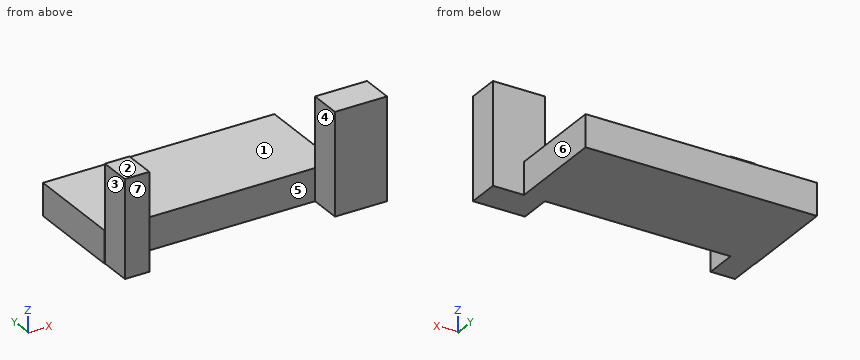
from build123d import *

# Parameters (mm, degrees)
F0_W     = 182.7251240611
F0_H     = 78.556381166
F1_DEPTH = 25.4
F2_W     = 19.2864239216
F2_H     = 76.4613673091
F3_DEPTH = 25.4
F4_W     = 15.6851392239
F4_H     = 80.182261765
F5_DEPTH = 25.4
F6_DEPTH = 25.4


with BuildPart() as f1:
    # F0 (on Top) → F1 (new body)
    with BuildSketch(Plane.XY):
        with Locations((-55.9463985264, 39.278190583)):
            Rectangle(F0_W, F0_H)
    extrude(amount=F1_DEPTH)

    # F2 (on Front) → F3 (join)
    with BuildSketch(Plane.XZ):
        with Locations((-137.3333185911, 38.2306836545)):
            Rectangle(F2_W, F2_H)
    extrude(amount=F3_DEPTH)

    # F4 (on Front) → F5 (join)
    with BuildSketch(Plane.XZ):
        with Locations((26.723430492, 40.0911308825)):
            Rectangle(F4_W, F4_H)
    extrude(amount=F5_DEPTH)

    # F6 (add): a face of the model
    f6_faces = [f1.faces().sort_by_distance(p)[0] for p in [
        (34.566000104, -12.7, 40.0911308825),
    ]]
    extrude(f6_faces, amount=F6_DEPTH)


solid = f1.part
Geometry check sheet. Reference: the model listing, model coordinates, mm. Face numbers are marked on the shaded views. A direction names the side the tool comes from. Round coordinates to 2 decimals unless told otherwise and drop trailing zeros. Order: outer loops, then holes, each group sorted by start corner. A loop starts at its lowest first (then second) coordinate and runs counter-clockwise, first axis right, second up. Notation, with made-up numbers: (37.25, 65) -> (65.25, 65) arc R17 ccw to (65.25, 90) -> close; hole circle Ø9 at (-22, 52.25). An arc over 180 degrees is marked (long way). Use one line per item in the form item = value.
1. Cross-section at C-C, the plane x = 22.5. Enter the section's corners in (y, z).
Working result:
outline = (-25.4, 0) -> (78.56, 0) -> (78.56, 25.4) -> (0, 25.4) -> (0, 80.18) -> (-25.4, 80.18) -> close
2. Go/stop test with flat-tipped pins: pin 1 (20.5 mm diameter, centred on y = -15, z = 42.5, fed in from -X); pin 2 (12.5 mm diameter, centred on y = 47, z = 12, fed in from +X); pin 3 (6 mm diameter, centred on x = -134, z = 55.5, fed in from +Y). Record where each tip stops, or that it passes through.
Working result:
pin_1 = -146.98
pin_2 = 35.42
pin_3 = 0
3. Cross-section at B-B, the plane y = -2. Enter the section's corners in (x, z), plus the area to 3 significant figures.
Working result:
outline = (-146.98, 0) -> (-127.69, 0) -> (-127.69, 76.46) -> (-146.98, 76.46) -> close; (18.88, 0) -> (59.97, 0) -> (59.97, 80.18) -> (18.88, 80.18) -> close
area = 4,770 mm^2
4. Mould release check, pull along X, two halves, no side actions. Record for the marked faces 5, 6 and 7: pulls with the +X half, pulls with the -X half, needs draft (parallel to the pull), parting line crosses it, or undercut.
Working result:
face_5 = undercut
face_6 = pulls with the +X half
face_7 = needs draft
5. Cross-section at A-A, the plane z = 40.5. Enter the section's corners in (x, y), plus the area to 3 significant figures.
Working result:
outline = (-146.98, -25.4) -> (-127.69, -25.4) -> (-127.69, 0) -> (-146.98, 0) -> close; (18.88, -25.4) -> (59.97, -25.4) -> (59.97, 0) -> (18.88, 0) -> close
area = 1,530 mm^2
6. Cross-section at D-D, the plane z = 9. Enter the section's corners in (x, y).
Working result:
outline = (-147.31, 0) -> (-146.98, 0) -> (-146.98, -25.4) -> (-127.69, -25.4) -> (-127.69, 0) -> (18.88, 0) -> (18.88, -25.4) -> (59.97, -25.4) -> (59.97, 0) -> (35.42, 0) -> (35.42, 78.56) -> (-147.31, 78.56) -> close
7. Set-up check for the marked faces 1, 2, 3 and 4: record each of +Z, -Z, +X, -X, +Y, -Y from which the full face is reachable in a straight line by a thin tool's end or side.
Working result:
face_1 = +Z, +X, -X, +Y
face_2 = +Z, -X, +Y, -Y
face_3 = +Z, -Z, -X, -Y
face_4 = +Z, -Z, -Y
8. Scan lines: line 1 along X through (y, z) = (-10, 34); line 2 along Y through (x, z) = (34.5, 62.5); line 3 along Z through (x, y) = (28, 13.5). Record each from-to range of solid material in increasing order. Write a range as from..to.
Working result:
line_1 = -146.98..-127.69, 18.88..59.97
line_2 = -25.4..0
line_3 = 0..25.4
